from build123d import *

# Parameters (mm, degrees)
SKETCH1_R           = 1
BOSS_EXTRUDE1_DEPTH = 1.5
FILLET1_R           = 3
CUT_EXTRUDE1_DEPTH  = 79.931932702
LPATTERN1_COUNT     = 16
LPATTERN1_PITCH     = 3
CUT_EXTRUDE2_DEPTH  = 79.931932702
FILLET2_R           = 0.3
CUT_EXTRUDE3_DEPTH  = 5
FILLET3_R           = 0.808139
FILLET4_R           = 0.823652
CUT_EXTRUDE4_DEPTH  = 1.6
FILLET10_R          = 1
FILLET11_R          = 0.5
FILLET13_R          = 3.7
FILLET14_R          = 2.2


with BuildPart() as part:
    # Sketch1 → Boss-Extrude1 (new body)
    with BuildSketch(Plane(origin=(0, 0, 0), x_dir=(1, 0, 0), z_dir=(0, 1, 0))):
        Polygon((0, 0), (0, 6), (1, 78), (6, 78), (9, 18), (12, 18), (10, 0), align=None)
        with Locations(Location((8, 8, 0), (0, 0, 270))):
            Circle(SKETCH1_R, mode=Mode.SUBTRACT)
    extrude(amount=BOSS_EXTRUDE1_DEPTH)

    # Fillet1
    fillet1_edges = [part.edges().sort_by_distance(p)[0] for p in [
        (10, 0.75, 0),
    ]]
    fillet(fillet1_edges, radius=FILLET1_R)

    # Sketch2 → Cut-Extrude1 (cut, symmetric)
    with BuildSketch(Plane(origin=(0, 1.5, 0), x_dir=(1, 0, 0), z_dir=(0, 1, 0))):
        with BuildLine():
            ThreePointArc((4.955729038, 71.878708516), (4.750594632, 71.450097336), (4.996498521, 71.04350301))
            Line((4.996498521, 71.04350301), (6.194975811, 70.338548499))
            ThreePointArc((6.194975811, 70.338548499), (6.340221232, 70.195153453), (6.4, 70))
            Line((6.4, 70), (6.25, 73))
            ThreePointArc((6.25, 73), (6.19798995, 72.829948537), (6.079849196, 72.697037636))
            Line((6.079849196, 72.697037636), (4.955729038, 71.878708516))
        make_face()
    cut_extrude1 = extrude(amount=CUT_EXTRUDE1_DEPTH, both=True, mode=Mode.SUBTRACT)

    # LPattern1: Cut-Extrude1 ×16
    with Locations(*[Vector(0.0499376169438922, 0, 0.9987523388778448) * (i * LPATTERN1_PITCH) for i in range(1, LPATTERN1_COUNT)]):
        add(cut_extrude1, mode=Mode.SUBTRACT)

    # Sketch3 → Cut-Extrude2 (cut, through all)
    with BuildSketch(Plane(origin=(0, 1.5, 0), x_dir=(1, 0, 0), z_dir=(0, 1, 0))):
        with BuildLine():
            Line((8.496742185, 24.698632232), (6.822120402, 21.727534299))
            ThreePointArc((6.822120402, 21.727534299), (6.841431522, 19.238817172), (9, 18))
            Line((9, 18), (8.647192762, 25.05614475))
            ThreePointArc((8.647192762, 25.05614475), (8.608047789, 24.862204955), (8.496742185, 24.698632232))
        make_face()
    extrude(amount=-CUT_EXTRUDE2_DEPTH, mode=Mode.SUBTRACT)

    # Fillet2
    fillet2_edges = [part.edges().sort_by_distance(p)[0] for p in [
        (12, 0.75, -18),
    ]]
    fillet(fillet2_edges, radius=FILLET2_R)

    # Sketch16 → Cut-Extrude3 (cut)
    with BuildSketch(Plane.XZ):
        with BuildLine():
            Line((6, -78), (4.5, -78))
            Line((4.5, -78), (4.292293166, -76.514450313))
            ThreePointArc((4.292293166, -76.514450313), (3.5, -75.825227292), (2.707706834, -76.514450313))
            Line((2.707706834, -76.514450313), (2.5, -78))
            Line((2.5, -78), (1, -78))
            Line((1, -78), (1, -78.416520576))
            Line((1, -78.416520576), (6, -78.416520576))
            Line((6, -78.416520576), (6, -78))
        make_face()
    extrude(amount=-CUT_EXTRUDE3_DEPTH, mode=Mode.SUBTRACT)

    # Fillet3
    fillet3_edges = [part.edges().sort_by_distance(p)[0] for p in [
        (1, 0.75, -78),
        (2.5, 0.75, -78),
    ]]
    fillet(fillet3_edges, radius=FILLET3_R - 0.0001)  # a hair under: the kernel refuses the full size

    # Fillet4
    fillet4_edges = [part.edges().sort_by_distance(p)[0] for p in [
        (6, 0.75, -78),
        (4.5, 0.75, -78),
    ]]
    fillet(fillet4_edges, radius=FILLET4_R - 0.0001)  # a hair under: the kernel refuses the full size

    # Sketch15 → Cut-Extrude4 (cut)
    with BuildSketch(Plane(origin=(0, 1.5, 0), x_dir=(1, 0, 0), z_dir=(0, 1, 0))):
        Polygon((4.2, 14.9), (4.2, 4.2), (11.363579638, 4.2), (10.97286707, 0), (4.2, 0), (0, 0), (0, 14.9), align=None)
    extrude(amount=-CUT_EXTRUDE4_DEPTH, mode=Mode.SUBTRACT)

    # Fillet10
    fillet10_edges = [part.edges().sort_by_distance(p)[0] for p in [
        (0.123611111, 0.75, -14.9),
    ]]
    fillet(fillet10_edges, radius=FILLET10_R)

    # Fillet11
    fillet11_edges = [part.edges().sort_by_distance(p)[0] for p in [
        (4.2, 0.75, -14.9),
    ]]
    fillet(fillet11_edges, radius=FILLET11_R)

    # Fillet13
    fillet13_edges = [part.edges().sort_by_distance(p)[0] for p in [
        (4.2, 0.75, -4.2),
    ]]
    fillet(fillet13_edges, radius=FILLET13_R)

    # Fillet14
    fillet14_edges = [part.edges().sort_by_distance(p)[0] for p in [
        (10.466666667, 0.75, -4.2),
    ]]
    fillet(fillet14_edges, radius=FILLET14_R)


solid = part.part
Geometry check sheet. Reference: the model listing, model coordinates, mm. A direction names the side the tool comes from. Coordinates: 2 decimals unless noted, no trailing zeros. Loops run counter-clockwise (first coordinate to the right, second up) from the corner with the lowest first, then second, coordinate; pieces in that order, holes last. Notation, with made-up numbers: (19.25, 89.5) - (61.25, 89.5) arc R27 ccw to (61.25, 119.5) - close; hole circle Ø10 at (23, 17.5). An arc over 180 degrees is marked (long way). Use one line per item in the form item = value. Start each with the question number.
Item 1: Thickness scan on probe 1 along X at (y, z) = (0.5, -8); probe 2 along X at (y, z) = (0.55, -21); probe 3 along Z at (x, y) = (10.25, 0.5). Record the ranges inside material, lowest first.
Item 2: Tool access check on faces 1 (the face through (5.68, 0.76, -69.3)), 2 (the face through (2, 1, -14.9)). Record the directions out of +Z, -Z, +X, -X, +Y, -Y that give a thin tool (end or side, any length) a straight path to the whole face; none if there is none.
Item 3: Gauge pin test, flat end, axial feed: pin 1 (0.8 mm diameter, centred on y = 0.5, z = -9.5, fed in from -X). Record the tip position at first contact, or that the pin passes through.
Item 4: Mould release check, pull along Z, two halves, no side actions. Record for faces 3 (the face through (5, 0, -42)), 4 (the face through (11.333, 0.74, -11.993)), 5 (the face through (6.64, 0.76, -49.72)): +Z half, -Z half, draft (parallel to the pull), parting line (faces both ways), or undercut.
Item 5: Section check A-A, the plane z = -13.5. Enter the section's corners in (x, y).
Computed:
q1.probe_1 = 4.2 to 7, 9 to 10.89
q1.probe_2 = 0.21 to 6.55
q1.probe_3 = -18 to -5.07
q2.face_1 = +X, +Y, -Y
q2.face_2 = +Z, -X, +Y, -Y
q3.pin_1 = 4.2
q4.face_3 = draft
q4.face_4 = +Z half
q4.face_5 = undercut
q5.outline = (4.2, 0) - (11.5, 0) - (11.5, 1.5) - (4.2, 1.5) - close
